Here's how the part is built. I have some questions about the finished solid (model axes, mm). Round coordinates to 2 decimals unless told otherwise and drop trailing zeros. Loops run counter-clockwise (first coordinate to the right, second up) from the corner with the lowest first, then second, coordinate; pieces in that order, holes last. Notation, with made-up numbers: M 72,-23.75 L 94,-23.75 A12 cw 94,-7.75 Z; hole C 40,70.5 d1. An arc over 180 degrees is marked long. Answer as a JSON object with one key per item and string values.
from build123d import *

# Parameters (mm, degrees)
SKETCH_W             = 254
SKETCH_H             = 57.15
PAD_DEPTH            = 31.75
POCKET_DEPTH         = 31.751
FILLET_R             = 12.7
SKETCH002_R          = 11.1125
POCKET001_DEPTH      = 127.001
POCKET001_DEPTH_BACK = -127.001


with BuildPart() as part:
    # Sketch → Pad (new body)
    with BuildSketch(Plane.XY):
        Rectangle(SKETCH_W, SKETCH_H)
    extrude(amount=PAD_DEPTH)

    # Sketch001 (on Face6 of Pad) → Pocket (cut, through all)
    with BuildSketch(Plane.XY.offset(31.75)):
        with BuildLine():
            ThreePointArc((-98.425, 28.575), (-127, 0), (-98.425, -28.575))
            Line((-98.425, -28.575), (-145.596313, -28.575))
            Line((-145.596313, 28.575), (-145.596313, -28.575))
            Line((-98.425, 28.575), (-145.596313, 28.575))
        make_face()
        with BuildLine():
            ThreePointArc((98.425, -28.575), (127, 0), (98.425, 28.575))
            Line((98.425, 28.575), (145.596313, 28.575))
            Line((145.596313, 28.575), (145.596313, -28.575))
            Line((98.425, -28.575), (145.596313, -28.575))
        make_face()
    extrude(amount=-POCKET_DEPTH, mode=Mode.SUBTRACT)

    # Fillet
    fillet_edges = [part.edges().sort_by_distance(p)[0] for p in [
        (-118.630576, -20.205576, 31.75),
        (-118.630576, 20.205576, 31.75),
        (0, 28.575, 31.75),
        (118.630576, 20.205576, 31.75),
        (118.630576, -20.205576, 31.75),
        (0, -28.575, 31.75),
    ]]
    fillet(fillet_edges, radius=FILLET_R)

    # Sketch002 → Pocket001 (cut, two sides)
    with BuildSketch(Plane.YZ) as pocket001_sk:
        with Locations((0, -6.35)):
            Circle(SKETCH002_R)
    extrude(amount=-POCKET001_DEPTH, mode=Mode.SUBTRACT)
    extrude(pocket001_sk.sketch, amount=-POCKET001_DEPTH_BACK, mode=Mode.SUBTRACT)


solid = part.part
Item 1: I want a section at C-C on z = 9. List the corners of the cut face in (x, y) for me (3 decimals).
Solution:
{"outline": "M -98.425,-28.575 L 98.425,-28.575 A28.575 ccw 98.425,28.575 L -98.425,28.575 A28.575 ccw Z"}
Item 2: For P1, Ø3, axis at x = -74.5, y = 9.5, coming from the -Z side; P2, Ø1, axis at x = 47.5, y = -8.5, coming from the -Z side; P3, Ø8, axis at x = -4, z = 25.5, coming from the +Y side; P4, Ø1.5, axis at y = -9, z = 26, coming from the +X side, each with a flat end and sliding along its axis, tell me the tip position at first contact or that it passes through.
Solution:
{"P1": "stops at z = 0", "P2": "stops at z = 0.17", "P3": "stops at y = 28.34", "P4": "stops at x = 123.91"}
Item 3: We'd pull the mould along Y, two halves only. Please class faces 1 (the face through (126.993, -0.628, 9.658)), 2 (the face through (-2, 0, 31.75)), 3 (the face through (1.78, 0.15, 4.76)): +Y half, -Y half, draft (parallel to the pull), parting line (faces both ways), or undercut.
Solution:
{"face 1": "parting line", "face 2": "draft", "face 3": "undercut"}
Item 4: If I drill on L1, parallel to X at y = 9, z = 19; L2, parallel to Z at x = -34.5, y = -0.5; L3, parallel to Z at x = 85, y = 16.5, over which ranges is the centre line in solid material (lowest first)? Write a range as from..to.
Solution:
{"L1": "x = -125.55..125.55", "L2": "z = 4.75..31.75", "L3": "z = 0..31.73"}
Item 5: I want a section at B-B on y = 0. List the corners of the cut face in (x, z) for me, plus the area to 3 significant figures.
Solution:
{"outline": "M -127,4.76 L 127,4.76 L 127,19.05 A12.7 ccw 114.3,31.75 L -114.3,31.75 A12.7 ccw -127,19.05 Z", "area": "6,790 mm2"}
